```python
from build123d import *

# Parameters (mm, degrees)
SALIENTE_EXTRUIR1_DEPTH = 50
CORTAR_EXTRUIR1_REACH   = 70.92
CROQUIS2_R              = 3.175


with BuildPart() as part:
    # Croquis1 → Saliente-Extruir1 (new body)
    with BuildSketch(Plane.XY):
        with BuildLine():
            Line((0, 0), (0, 9))
            Line((0, 9), (0, 18))
            ThreePointArc((0, 18), (-0.585786438, 19.414213562), (-2, 20))
            Line((-2, 20), (-8.5, 20))
            Line((-8.5, 20), (-15, 20))
            Line((-15, 20), (-15, 15))
            Line((-15, 15), (-5, 15))
            Line((-5, 15), (-5, 0))
            Line((-5, 0), (-5, -23))
            ThreePointArc((-5, -23), (-4.414213562, -24.414213562), (-3, -25))
            Line((-3, -25), (10, -25))
            Line((10, -25), (10, -20))
            Line((10, -20), (0, -20))
            Line((0, -20), (0, 0))
        make_face()
    extrude(amount=SALIENTE_EXTRUIR1_DEPTH)

    # Croquis2 → Cortar-Extruir1 (cut, up to next)
    with BuildSketch(Plane.XZ.offset(25), mode=Mode.PRIVATE) as cortar_extruir1_sk1:
        with Locations(Location((5, 25, 0), (0, 0, 270))):
            Circle(CROQUIS2_R)
    cortar_extruir1_tool1 = extrude(cortar_extruir1_sk1.sketch, amount=-CORTAR_EXTRUIR1_REACH, mode=Mode.PRIVATE) & part.part
    add(cortar_extruir1_tool1.solids().sort_by_distance((5, -25, 25))[0], mode=Mode.SUBTRACT)


solid = part.part
```
Check sheet for the modelled part. Datum: model origin and axes. Units: mm. A direction names the side the tool comes from. Give positions to 0.01 mm unless a question says otherwise; leave off trailing zeros. Order: outer loops, then holes, each group sorted by start corner. A loop starts at its lowest first (then second) coordinate and runs counter-clockwise, first axis right, second up. Notation, with made-up numbers: M 10.25,16.25 L 38.25,16.25 A9 cw 38.25,32.25 Z; hole C 37.5,-32 d11. An arc over 180 degrees is marked long. Answer in a Markdown table with one row per item. Add a question column.
Q1. Access from +Z, -Z, +X, -X, +Y, -Y to the whole of each face (thin tool, end or side, straight path). Record for faces 1 (the flat face through (-10, 15, 25)), 2 (the flat face through (8.4, -20, 24.6)), 3 (the flat face through (-8, 20, 25)).
Q2. Sectioned sample at A-A, the plane z = 25. Record the boundary of the cut face in (x, y) (3 decimals).
Q3. Sectioned sample at B-B, the plane x = 5. Record the boundary of the cut face in (y, z) (3 decimals).
Q4. Release check for a two-part mould opening along Z. For faces 4 (the flat face through (-3, -1, 50)), 5 (the flat face through (-15, 18, 25)), 6 (the cylindrical face through (5.14, -22.54, 28.17)) record: released by +Z, released by -Z, zero draft, split by the parting line, or undercut.
Q5. Thickness scan on L1, parallel to X at y = -22.35, z = 25 (3 decimals); L2, parallel to Y at x = 5.5, z = 12; L3, parallel to Y at x = -5.75, z = 14. Record the ranges inside material, lowest first.
Q6. Gauge pin test, flat ends, axial feed: pin 1 Ø10 at (y, z) = (-19.5, 28) entering from -X; pin 2 Ø5 at (x, z) = (-5.5, 28.5) entering from -Y; pin 3 Ø1.5 at (y, z) = (2.5, 9.5) entering from +X; pin 4 Ø5.5 at (x, z) = (5, 25) entering from -Y. Record the tip position at first contact, or that the pin passes through.
Q7. Sectioned sample at C-C, the plane z = 10. Record the boundary of the cut face in (x, y).
Q8. Sectioned sample at D-D, the plane x = 1. Record the boundary of the cut face in (y, z).
Verdict:
| question | item | result |
|---|---|---|
| 1 | face 1 | +Z, -Z, -X, -Y |
| 1 | face 2 | +Z, -Z, +X, +Y |
| 1 | face 3 | +Z, -Z, +X, -X, +Y |
| 2 | outline | M -15,15 L -5,15 L -5,-23 A2 ccw -3,-25 L 1.825,-25 L 1.825,-20 L 0,-20 L 0,18 A2 ccw -2,20 L -15,20 Z; M 8.175,-25 L 10,-25 L 10,-20 L 8.175,-20 Z |
| 3 | outline | M -25,0 L -20,0 L -20,21.825 L -25,21.825 Z; M -25,28.175 L -20,28.175 L -20,50 L -25,50 Z |
| 4 | face 4 | released by +Z |
| 4 | face 5 | zero draft |
| 4 | face 6 | undercut |
| 5 | L1 | -5 to 1.825, 8.175 to 10 |
| 5 | L2 | -25 to -20 |
| 5 | L3 | 15 to 20 |
| 6 | pin 1 | x = -5 |
| 6 | pin 2 | y = -25 |
| 6 | pin 3 | x = 0 |
| 6 | pin 4 | through |
| 7 | outline | M -15,15 L -5,15 L -5,-23 A2 ccw -3,-25 L 10,-25 L 10,-20 L 0,-20 L 0,18 A2 ccw -2,20 L -15,20 Z |
| 8 | outline | M -25,0 L -20,0 L -20,50 L -25,50 Z |
